from build123d import *

# Parameters (mm, degrees)
F1_DEPTH = 3.175
F2_D     = 3.4544
F2_DEPTH = 21.43125
F2_TIP   = 1.0378064612
F3_D     = 4.318
F3_DEPTH = 15.875
F3_TIP   = 1.2972580765


with BuildPart() as f1:
    # F0 (on Right) → F1 (new body)
    with BuildSketch(Plane.YZ):
        with BuildLine():
            Line((16.1557392643, -17.4625), (12.7, -17.4625))
            Line((12.7, -17.4625), (12.7, -52.986030559))
            Line((12.7, -52.986030559), (34.5102887852, -48.6771610688))
            Line((34.5102887852, -48.6771610688), (34.5102887852, -30.4380403067))
            ThreePointArc((34.5102887852, -30.4380403067), (33.8915652541, -27.7040011635), (32.1559675137, -25.5027539424))
            Line((32.1559675137, -25.5027539424), (22.225, -17.4625))
            Line((22.225, -17.4625), (16.1557392643, -17.4625))
        make_face()
    extrude(amount=F1_DEPTH)

    # F2
    with Locations(Plane(origin=(0, 0, 0), x_dir=(0, 1, 0), z_dir=(-1, 0, 0))):
        with Locations((28.1602887852, 30.4380403067)):
            Hole(F2_D / 2, depth=F2_DEPTH)
            with Locations((0, 0, -(F2_DEPTH + F2_TIP / 2))):  # 118° drill point
                Cone(0, F2_D / 2, F2_TIP, mode=Mode.SUBTRACT)

    # F3
    with Locations(Plane(origin=(0, 0, 0), x_dir=(0, 1, 0), z_dir=(-1, 0, 0))):
        with Locations((17.4625, 22.225), (17.4625, 47.625)):
            Hole(F3_D / 2, depth=F3_DEPTH)
            with Locations((0, 0, -(F3_DEPTH + F3_TIP / 2))):  # 118° drill point
                Cone(0, F3_D / 2, F3_TIP, mode=Mode.SUBTRACT)


solid = f1.part
Here's how the part is built. I have some questions about the finished solid (model axes, mm). Coordinates: 2 decimals unless noted, no trailing zeros. Order: outer loops, then holes, each group sorted by start corner. A loop starts at its lowest first (then second) coordinate and runs counter-clockwise, first axis right, second up.
Item 1: If we section it at C-C on y = 19: List the corners of the cut face in (x, z) for me (1 decimal).
Result sheet:
outline: (0, -51.7) - (3.2, -51.7) - (3.2, -49.1) - (0, -49.1) - close; (0, -46.1) - (3.2, -46.1) - (3.2, -23.7) - (0, -23.7) - close; (0, -20.7) - (3.2, -20.7) - (3.2, -17.5) - (0, -17.5) - close
Item 2: If we section it at B-B on y = 28.75: List the corners of the cut face in (x, z) for me (3 decimals), plus the area to 3 significant figures.
Result sheet:
outline: (0, -49.815) - (3.175, -49.815) - (3.175, -32.061) - (0, -32.061) - close; (0, -28.815) - (3.175, -28.815) - (3.175, -22.745) - (0, -22.745) - close
area: 75.6 mm2
Item 3: If we section it at A-A on z = -23: List the corners of the cut face in (x, y) for me (3 decimals), plus the area to 3 significant figures.
Result sheet:
outline: (0, 12.7) - (3.175, 12.7) - (3.175, 15.447) - (0, 15.447) - close; (0, 19.478) - (3.175, 19.478) - (3.175, 29.065) - (0, 29.065) - close
area: 39.2 mm2
Item 4: For P1, Ø3, axis at y = 28.16, z = -30.44, coming from the -X side, with a flat end and sliding along its axis, tell me the tip position at first contact or that it passes through.
Result sheet:
P1: passes through
Item 5: I need wall thicknesses on line 1 (Z direction, x = 2.3, y = 18); line 2 (Y direction, x = 2.6, z = -30); line 3 (Z direction, x = 0.8, y = 27). Which ranges of each line are inside material? Lowest first, please.
Result sheet:
line 1: z = -51.94 to -49.72, -45.53 to -24.32, -20.13 to -17.46
line 2: y = 12.7 to 26.49, 29.83 to 34.5
line 3: z = -50.16 to -31.72, -29.16 to -21.33
Item 6: If we mould it in two halves opening along Z, with no side actions, what happens to faces 1 (the face through (1.565, 23.452, -50.862)), 2 (the face through (1.61, 17.744, -24.366)), 3 (the face through (2, 34.51, -40))? For each: +Z half, -Z half, draft (parallel to the pull), parting line (faces both ways), or undercut.
Result sheet:
face 1: -Z half
face 2: undercut
face 3: draft
Item 7: If we section it at D-D on x = 1: State how many separate pieces and enclosed holes the cut face has, plus the area to 3 significant figures.
Result sheet:
separate pieces: 1
enclosed holes: 3
area: 627 mm2
